```python
from build123d import *

# Parameters (mm, degrees)
BOSS_EXTRUDE1_DEPTH   = 550
F_4_0MM_DOWEL_HOLE1_D = 4
CUT_EXTRUDE1_DEPTH    = 579.75873098
SKETCH7_W             = 100
SKETCH7_H             = 409.5
CUT_EXTRUDE2_DEPTH    = 575.598945437
SKETCH8_W             = 100
SKETCH8_H             = 2
BOSS_EXTRUDE2_DEPTH   = 23
SKETCH9_W             = 100
SKETCH9_H             = 2
BOSS_EXTRUDE3_DEPTH   = 364
SKETCH10_W            = 100
SKETCH10_H            = 64.953820437
CUT_EXTRUDE3_DEPTH    = 364
SKETCH11_W            = 100
SKETCH11_H            = 35.696147614
CUT_EXTRUDE4_DEPTH    = 364
SKETCH12_W            = 5
SKETCH12_H            = 4
CUT_EXTRUDE6_DEPTH    = 575.781517842
SKETCH13_W            = 35
SKETCH13_H            = 2
CUT_EXTRUDE7_DEPTH    = 575.781517842
BOSS_EXTRUDE4_DEPTH   = 2
SKETCH15_W            = 35
SKETCH15_H            = 2
CUT_EXTRUDE8_DEPTH    = 575.781517842
SKETCH18_W            = 100
SKETCH18_H            = 7.149859065
CUT_EXTRUDE10_DEPTH   = 73.5
SKETCH22_W            = 2
SKETCH22_H            = 28
BOSS_EXTRUDE8_DEPTH   = 364
SKETCH24_W            = 2
SKETCH24_H            = 28
BOSS_EXTRUDE9_DEPTH   = 364


with BuildPart() as part:
    # Sketch1 → Boss-Extrude1 (new body)
    with BuildSketch(Plane.XY):
        Polygon((-165.647058824, 7.852941176), (-165.647058824, -7.147058824), (14.352941176, -7.147058824), (14.352941176, 7.852941176), (9.352941176, 7.852941176), (9.352941176, -2.147058824), (-160.647058824, -2.147058824), (-160.647058824, 7.852941176), align=None)
    extrude(amount=BOSS_EXTRUDE1_DEPTH)

    # Ø4.0mm Dowel Hole1 (through all)
    with Locations(Plane(origin=(14.352941176, 0, 0), x_dir=(0, 0, -1), z_dir=(1, 0, 0))):
        with Locations((-540, -0.147058824)):
            Hole(F_4_0MM_DOWEL_HOLE1_D / 2)

    # Sketch5 → Cut-Extrude1 (cut, through all)
    with BuildSketch(Plane(origin=(14.352941176, 0, 0), x_dir=(0, 0, -1), z_dir=(1, 0, 0))):
        with BuildLine():
            Line((-65, 1.852941176), (-15, 1.852941176))
            ThreePointArc((-15, 1.852941176), (-13, -0.147058824), (-15, -2.147058824))
            Line((-15, -2.147058824), (-65, -2.147058824))
            ThreePointArc((-65, -2.147058824), (-67, -0.147058824), (-65, 1.852941176))
        make_face()
    extrude(amount=-CUT_EXTRUDE1_DEPTH, mode=Mode.SUBTRACT)

    # Sketch7 → Cut-Extrude2 (cut, through all)
    with BuildSketch(Plane.XZ.offset(7.147058824)):
        with Locations((-75.647058824, 269.75)):
            Rectangle(SKETCH7_W, SKETCH7_H)
    extrude(amount=-CUT_EXTRUDE2_DEPTH, mode=Mode.SUBTRACT)

    # Sketch8 → Boss-Extrude2 (add)
    with BuildSketch(Plane(origin=(0, -2.147058824, 0), x_dir=(1, 0, 0), z_dir=(0, 1, 0))):
        with Locations((-75.647058824, -475.5)):
            Rectangle(SKETCH8_W, SKETCH8_H)
    extrude(amount=BOSS_EXTRUDE2_DEPTH)

    # Sketch9 → Boss-Extrude3 (add)
    with BuildSketch(Plane(origin=(0, 0, 474.5), x_dir=(-1, 0, 0), z_dir=(0, 0, -1))):
        with Locations((75.647058824, 19.852941176)):
            Rectangle(SKETCH9_W, SKETCH9_H)
    extrude(amount=BOSS_EXTRUDE3_DEPTH)

    # Sketch10 → Cut-Extrude3 (cut)
    with BuildSketch(Plane.XZ.offset(7.147058824)):
        with Locations((-75.647058824, 32.523089781)):
            Rectangle(SKETCH10_W, SKETCH10_H)
    extrude(amount=-CUT_EXTRUDE3_DEPTH, mode=Mode.SUBTRACT)

    # Sketch11 → Cut-Extrude4 (cut)
    with BuildSketch(Plane.XZ.offset(7.147058824)):
        with Locations((-75.647058824, -10.567416996)):
            Rectangle(SKETCH11_W, SKETCH11_H)
    extrude(amount=-CUT_EXTRUDE4_DEPTH, mode=Mode.SUBTRACT)

    # Sketch12 → Cut-Extrude6 (cut, through all)
    with BuildSketch(Plane(origin=(0, 0, 0), x_dir=(-1, 0, 0), z_dir=(0, 0, -1))):
        with Locations((-11.852941176, 5.852941176)):
            Rectangle(SKETCH12_W, SKETCH12_H)
        with Locations((163.147058824, 5.852941176)):
            Rectangle(SKETCH12_W, SKETCH12_H)
    extrude(amount=-CUT_EXTRUDE6_DEPTH, mode=Mode.SUBTRACT)

    # Sketch13 → Cut-Extrude7 (cut, through all)
    with BuildSketch(Plane(origin=(0, 0, 0), x_dir=(-1, 0, 0), z_dir=(0, 0, -1))):
        with Locations((8.147058824, -3.147058824)):
            Rectangle(SKETCH13_W, SKETCH13_H)
        with Locations((143.147058824, -3.147058824)):
            Rectangle(SKETCH13_W, SKETCH13_H)
    extrude(amount=-CUT_EXTRUDE7_DEPTH, mode=Mode.SUBTRACT)

    # Sketch14 → Boss-Extrude4 (add)
    with BuildSketch(Plane.XZ.offset(7.147058824)):
        Polygon((-165.647058824, 0), (-125.647058824, 0), (-125.647058824, 474.5), (-25.647058824, 474.5), (-25.647058824, 0), (14.352941176, 0), (14.352941176, 550), (-165.647058824, 550), align=None)
    extrude(amount=BOSS_EXTRUDE4_DEPTH)

    # Sketch15 → Cut-Extrude8 (cut, through all)
    with BuildSketch(Plane(origin=(0, 0, 0), x_dir=(-1, 0, 0), z_dir=(0, 0, -1))):
        with Locations((143.147058824, -5.147058824)):
            Rectangle(SKETCH15_W, SKETCH15_H)
        with Locations((8.147058824, -5.147058824)):
            Rectangle(SKETCH15_W, SKETCH15_H)
    extrude(amount=-CUT_EXTRUDE8_DEPTH, mode=Mode.SUBTRACT)

    # Sketch18 → Cut-Extrude10 (cut)
    with BuildSketch(Plane.XY.offset(550)):
        with Locations((-75.647058824, -2.572129292)):
            Rectangle(SKETCH18_W, SKETCH18_H)
    extrude(amount=-CUT_EXTRUDE10_DEPTH, mode=Mode.SUBTRACT)

    # Sketch22 → Boss-Extrude8 (add)
    with BuildSketch(Plane(origin=(0, 0, 474.5), x_dir=(-1, 0, 0), z_dir=(0, 0, -1))):
        with Locations((124.647058824, 4.852941176)):
            Rectangle(SKETCH22_W, SKETCH22_H)
    extrude(amount=BOSS_EXTRUDE8_DEPTH)

    # Sketch24 → Boss-Extrude9 (add)
    with BuildSketch(Plane(origin=(0, 0, 474.5), x_dir=(-1, 0, 0), z_dir=(0, 0, -1))):
        with Locations((26.647058824, 4.852941176)):
            Rectangle(SKETCH24_W, SKETCH24_H)
    extrude(amount=BOSS_EXTRUDE9_DEPTH)


solid = part.part
```
Part model, mm, in its own coordinate system. A direction names the side the tool comes from. Coordinates: 2 decimals unless noted, no trailing zeros. Order: outer loops, then holes, each group sorted by start corner. A loop starts at its lowest first (then second) coordinate and runs counter-clockwise, first axis right, second up. Notation, with made-up numbers: (2.5, 52.5) - (16.5, 52.5) arc R10 cw to (16.5, 68.5) - close; hole circle Ø9 at (47.5, 40). An arc over 180 degrees is marked (long way). Return JSON: item names as keys, results as strings. Group by question number.
Item 1: Cut at A-A (z = 97.5). List the corners of the cut face in (x, y).
Item 2: Pull direction X, two halves, no side cores. Call faces 6 (the face through (-1, -7, 0)), 7 (the face through (-75, 18.853, 295)), 8 (the face through (14.353, -3, 271)): pulls with the +X half, pulls with the -X half, needs draft (parallel to the pull), parting line crosses it, or undercut.
Item 3: Cut at D-D (z = 497). List the corners of the cut face in (x, y).
Item 4: Cut at B-B (z = 418). List the corners of the cut face in (x, y).
Item 5: Which spindle directions (+Z, -Z, +X, -X, +Y, -Y) get a long thin tool onto all of the face, cutting with end or side? Do faces 1 (the face through (-123.647, 5, 295)), 2 (the face through (-60.6, 19.3, 110.5)), 3 (the face through (-76, 7, 476.5)), 4 (the face through (-75.2, -6.5, 550)), 5 (the face through (-125.647, 7, 296)). Say none if no direction does.
Item 6: Pin check, flat tips, straight feed: pin 1 (9 mm diameter, centred on x = -69.5, y = 4.5, fed in from -Z); pin 2 (4 mm diameter, centred on x = -73, z = 409.5, fed in from -Y); pin 3 (13.5 mm diameter, centred on x = -65.5, y = 5.5, fed in from +Z); pin 4 (8 mm diameter, centred on y = 7.5, z = 313.5, fed in from -X). Stop position of each tip, or through.
Item 7: Drill centre lines: probe 1 along X at (y, z) = (1.75, 440); probe 2 along X at (y, z) = (-6.5, 245); probe 3 along Y at (x, z) = (-164, 540). Where is each one in solid material? Low to high. Write a range as from..to.
Item 8: Cut at C-C (x = -116). List the corners of the cut face in (y, z), plus the area to 3 significant figures.
Check values:
{
 "1": {"outline": "(-165.65, -9.15) - (-125.65, -9.15) - (-125.65, -6.15) - (-160.65, -6.15) - (-160.65, 3.85) - (-165.65, 3.85) - close; (-25.65, -9.15) - (14.35, -9.15) - (14.35, 3.85) - (9.35, 3.85) - (9.35, -6.15) - (-25.65, -6.15) - close"},
 "2": {"face 6": "needs draft", "face 7": "undercut", "face 8": "pulls with the +X half"},
 "3": {"outline": "(-165.65, -9.15) - (14.35, -9.15) - (14.35, 3.85) - (9.35, 3.85) - (9.35, -6.15) - (-160.65, -6.15) - (-160.65, 3.85) - (-165.65, 3.85) - close"},
 "4": {"outline": "(-165.65, -9.15) - (-123.65, -9.15) - (-123.65, 18.85) - (-27.65, 18.85) - (-27.65, -9.15) - (14.35, -9.15) - (14.35, 3.85) - (9.35, 3.85) - (9.35, -6.15) - (-25.65, -6.15) - (-25.65, 20.85) - (-125.65, 20.85) - (-125.65, -6.15) - (-160.65, -6.15) - (-160.65, 3.85) - (-165.65, 3.85) - close"},
 "5": {"face 1": "-Z, -Y", "face 2": "-Z, +Y, -Y", "face 3": "+Z, +Y", "face 4": "+Z, +X, -X, +Y, -Y", "face 5": "+Z, -Z, +Y"},
 "6": {"pin 1": "stops at z = 474.5", "pin 2": "stops at y = 18.85", "pin 3": "stops at z = 476.5", "pin 4": "stops at x = -165.65"},
 "7": {"probe 1": "x = -165.65..-160.65, -125.65..-123.65, -27.65..-25.65, 9.35..14.35", "probe 2": "x = -165.65..-123.65, -27.65..14.35", "probe 3": "y = -9.15..-2.15, 1.85..3.85"},
 "8": {"outline": "(-9.15, 474.5) - (18.85, 474.5) - (18.85, 110.5) - (20.85, 110.5) - (20.85, 476.5) - (-6.15, 476.5) - (-6.15, 550) - (-9.15, 550) - close", "area": "1,010 mm2"}
}
